CAD build for the part. Positions are in the model's coordinates, mm. Coordinates: 2 decimals unless noted, no trailing zeros. Loops run counter-clockwise (first coordinate to the right, second up) from the corner with the lowest first, then second, coordinate; pieces in that order, holes last. Notation, with made-up numbers: (0, -16) -> (12, -16) arc R17 ccw to (12, -2) -> close; hole circle Ø7 at (-13, 88.25). An arc over 180 degrees is marked (long way). Answer as CSV lines item,"result". Start each with the question number.
Autodesk Inventor part; units mm, degrees
ref_plane "YZ Plane" through (0, 0, 0) normal (1, 0, 0) x (0, 1, 0)
ref_plane "XZ Plane" through (0, 0, 0) normal (0, 1, 0) x (-1, 0, 0)
ref_plane "XY Plane" through (0, 0, 0) normal (0, 0, 1) x (1, 0, 0)
sketch "草圖1" plane through (0, 0, 0) normal (0, 0, 1) x (1, 0, 0)
  line L0 (14.5, -21) -> (-14.5, -21)
  line L1 (-14.5, -21) -> (-14.5, 21)
  line L2 (-14.5, 21) -> (14.5, 21)
  line L3 (14.5, 21) -> (14.5, -21)
  line L4 (14.5, 21) -> (-14.5, -21) construction
  point P0 (0, 0)
  dimension "d0" = 29
  dimension "d1" = 42
extrude "擠出1" add sketch "草圖1" along normal blind 4
sketch "草圖2" plane through (0, 0, 4) normal (0, 0, 1) x (1, 0, 0)
  line L0 (9, -15.5) -> (-9, -15.5)
  line L1 (-9, -15.5) -> (-9, 15.5)
  line L2 (-9, 15.5) -> (9, 15.5)
  line L3 (9, 15.5) -> (9, -15.5)
  line L4 (9, 15.5) -> (-9, -15.5) construction
  point P0 (0, 0)
  dimension "d4" = 31
  dimension "d5" = 18
hole "孔1" at (-9, 15.5, 4) at (9, 15.5, 4) at (9, -15.5, 4) at (-9, -15.5, 4) direction (0, 0, -1) diameter 6 end through all
sketch "草圖3" plane through (0, 0, 4) normal (0, 0, 1) x (1, 0, 0)
  line L0 (-14.5, -21) -> (-14.5, 21)
  line L1 (14.5, -21) -> (-14.5, -21)
  line L2 (14.5, 21) -> (14.5, -21)
  line L3 (-14.5, -6.85) -> (14.5, -6.85)
  line L4 (14.5, -6.85) -> (14.5, -7.15)
  line L5 (14.5, -7.15) -> (-14.5, -7.15)
  line L6 (-14.5, -7.15) -> (-14.5, -6.85)
  line L7 (-14.5, 0.15) -> (14.5, 0.15)
  line L8 (14.5, 0.15) -> (14.5, -0.15)
  line L9 (14.5, -0.15) -> (-14.5, -0.15)
  line L10 (-14.5, -0.15) -> (-14.5, 0.15)
  line L11 (-14.5, -7) -> (14.5, -7)
  line L12 (-14.5, 0) -> (14.5, 0)
  point P0 (0, 0)
  dimension "d13" = 0.3
  dimension "d14" = 0.3
  dimension "d15" = 14
  dimension "d16" = 21
emboss "浮雕1" sketch "草圖3" operation cut depth 0.1 direction (0, 0, -1) contours L0 L11 L2 L5 | L0 L3 L2 L11 | L0 L12 L2 L9 | L0 L7 L2 L12
properties part number "EBARA A Type 馬達側油視窗" material "PMMA 塑膠"
Item 1: Saw through at B-B (x = -9). Write the cut outline in (y, z), plus the area to 3 significant figures.
Item 2: Two-plate mould, pull along X, no slides. Class faces 1 (the face through (14.5, 0, 2)), 2 (the face through (8.9, 18.5, 2)), 3 (the face through (-14.5, 0, 2)), 4 (the face through (0, 0, 0)): pulls with the +X half, pulls with the -X half, needs draft (parallel to the pull), parting line crosses it, or undercut.
Item 3: Flat gauge pin, fed straight in: pin 1 Ø5 at (x, y) = (-9, 15.5) entering from -Z. Where does the tip first touch, or does it go through?
Item 4: Wall check: probe 1 along Y at (x, z) = (9, 2); probe 2 along X at (y, z) = (-15.5, 2.55); probe 3 along Y at (x, z) = (11.5, 2.65). Give the ranges that are in metal, low to high.
Item 5: Saw through at A-A (y = 15.5). Write the cut outline in (x, z).
Item 6: Saw through at C-C (z = 1.85). Write the cut outline in (x, y), plus the area to 3 significant figures.
Geometry check:
1,outline,"(-21, 0) -> (-18.5, 0) -> (-18.5, 4) -> (-21, 4) -> close; (-12.5, 0) -> (12.5, 0) -> (12.5, 4) -> (0.15, 4) -> (0.15, 3.9) -> (-0.15, 3.9) -> (-0.15, 4) -> (-6.85, 4) -> (-6.85, 3.9) -> (-7.15, 3.9) -> (-7.15, 4) -> (-12.5, 4) -> close; (18.5, 0) -> (21, 0) -> (21, 4) -> (18.5, 4) -> close"
1,area,"120 mm2"
2,face 1,"pulls with the +X half"
2,face 2,"undercut"
2,face 3,"pulls with the -X half"
2,face 4,"needs draft"
3,pin 1,"through"
4,probe 1,"-21 to -18.5, -12.5 to 12.5, 18.5 to 21"
4,probe 2,"-14.5 to -12, -6 to 6, 12 to 14.5"
4,probe 3,"-21 to -17.16, -13.84 to 13.84, 17.16 to 21"
5,outline,"(-14.5, 0) -> (-12, 0) -> (-12, 4) -> (-14.5, 4) -> close; (-6, 0) -> (6, 0) -> (6, 4) -> (-6, 4) -> close; (12, 0) -> (14.5, 0) -> (14.5, 4) -> (12, 4) -> close"
6,outline,"(-14.5, -21) -> (14.5, -21) -> (14.5, 21) -> (-14.5, 21) -> close; hole circle Ø6 at (-9, -15.5); hole circle Ø6 at (-9, 15.5); hole circle Ø6 at (9, -15.5); hole circle Ø6 at (9, 15.5)"
6,area,"1,100 mm2"
